Could you check a few things on this model? Use its own coordinates, in mm. A direction names the side the tool comes from. Coordinates: 2 decimals unless noted, no trailing zeros. Loops run counter-clockwise (first coordinate to the right, second up) from the corner with the lowest first, then second, coordinate; pieces in that order, holes last. Notation, with made-up numbers: M 73.25,39 L 94.25,39 A26 cw 94.25,64 Z; hole C 23,48.5 d11. An arc over 180 degrees is marked long. Use one line per item in the form item = value. Start each with the question number.
Solid Edge part; units mm, degrees
sketch "Sketch1" plane through (0, 0, 0) normal (1, 0, 0) x (0, 1, 0)
  line L0 (0, 0) -> (0, 95)
  line L1 (0, 95) -> (100, 95)
  line L2 (100, 95) -> (100, 67)
  line L3 (100, 67) -> (68, 67)
  line L4 (68, 67) -> (68, 0)
  line L5 (0, 0) -> (68, 0)
extrude "Protrusion1" add sketch "Sketch1" against normal blind 8
hole "Hole_1" at (0, 33, 46) direction (-1, 0, 0) diameter 51 end through all
hole "Hole1" at (0, 54.9203, 24.0797) direction (-1, 0, 0) diameter 6.8 end through all
hole "Hole2" at (0, 11.0797, 67.9203) direction (-1, 0, 0) diameter 6.8 end through all
properties part number "88823"
Item 1: I want a section at A-A (z = 46). Write out the boundary of the cut face in (x, y).
Item 2: For faces 1 (the flat face through (-4, 68, 34)), 2 (the flat face through (0, 49, 69)), which set-ups out of +Z, -Z, +X, -X, +Y, -Y let a thin tool reach every point of the face, with its end or its side?
Item 3: I want a section at D-D (y = 84.5). Write out the boundary of the cut face in (x, z).
Item 4: Please list where these lines run through material, in increasing order: line 1 along Z through (x, y) = (-7.5, 11); line 2 along Z through (x, y) = (-3.5, 33); line 3 along Z through (x, y) = (-0.5, 12).
Item 5: Thinking about a two-plate mould opening in Y: for faces 3 (the cylindrical face through (-3.944, 40.66, 21.678)), 4 (the flat face through (-4, 84, 67)), 5 (the cylindrical face through (-3.944, 51.904, 22.511)), 6 (the flat face through (-4, 100, 81)), which applies, pulls with the +Y half, pulls with the -Y half, needs draft (parallel to the pull), parting line crosses it, or undercut?
Item 6: I want a section at C-C (x = -3.5). Write out the boundary of the cut face in (y, z).
Item 7: I want a section at B-B (y = 33). Write out the boundary of the cut face in (x, z), plus the area to 3 significant figures.
Item 8: I'm going to push flat-ended pins straight in: P1, Ø2, axis at x = -3.5, y = 73.5, coming from the -Z side; P2, Ø2.5, axis at x = -2, z = 36.5, coming from the +Y side. Where does each tip first touch, or does it pass through?
Worked answers:
q1.outline = M -8,0 L 0,0 L 0,7.5 L -8,7.5 Z; M -8,58.5 L 0,58.5 L 0,68 L -8,68 Z
q2.face_1 = -Z, +X, -X, +Y
q2.face_2 = +Z, -Z, +X, +Y, -Y
q3.outline = M -8,67 L 0,67 L 0,95 L -8,95 Z
q4.line_1 = 0 to 33.11, 58.89 to 64.52, 71.32 to 95
q4.line_2 = 0 to 20.5, 71.5 to 95
q4.line_3 = 0 to 31.53, 60.47 to 64.65, 71.19 to 95
q5.face_3 = undercut
q5.face_4 = needs draft
q5.face_5 = undercut
q5.face_6 = pulls with the +Y half
q6.outline = M 0,0 L 68,0 L 68,67 L 100,67 L 100,95 L 0,95 Z; hole C 33,46 d51; hole C 11.08,67.92 d6.8; hole C 54.92,24.08 d6.8
q7.outline = M -8,0 L 0,0 L 0,20.5 L -8,20.5 Z; M -8,71.5 L 0,71.5 L 0,95 L -8,95 Z
q7.area = 352 mm²
q8.P1 = 67
q8.P2 = 68
